Can you work these out from the model? Positions are in its coordinate system, mm. Round coordinates to 2 decimals unless told otherwise and drop trailing zeros. Write each loop counter-clockwise with the first axis right and the second up, starting at its lowest first coordinate (ties: lowest second). Pieces come first, ordered by that corner, then holes. Notation, with made-up numbers: (88.5, 36) - (140.5, 36) arc R35 ccw to (140.5, 75) - close; hole circle Ø3 at (66, 33.25). An arc over 180 degrees is marked (long way). One line per item, written item: value. Start each with the question number.
(1) I want a section at B-B on y = 0. List the corners of the cut face in (x, z) for me, plus the area to 3 significant figures.
(2) I want a section at D-D on z = -5. List the corners of the cut face in (x, y) for me.
(3) I want a section at A-A on z = 17.5. List the corners of the cut face in (x, y) for me, plus the area to 3 significant figures.
(4) I want a section at C-C on x = 0.9. List the corners of the cut face in (y, z) for me.
(5) I'm going to push flat-ended pins straight in: pin 1 Ø2 at (x, y) = (0, 0) entering from +Z; pin 2 Ø1.5 at (x, z) = (-0.5, 7) entering from -Y; pin 3 Ø1.2 at (x, y) = (0, -0.5) entering from -Z. Where does each tip first touch, or does it pass through?
(6) If I drill on L1, parallel to X at y = 0, z = 17.7; L2, parallel to Z at x = -0.4, y = 1; L3, parallel to Y at x = 0.8, z = 2.5, over which ranges is the centre line in solid material (lowest first)? Write a range as from..to.
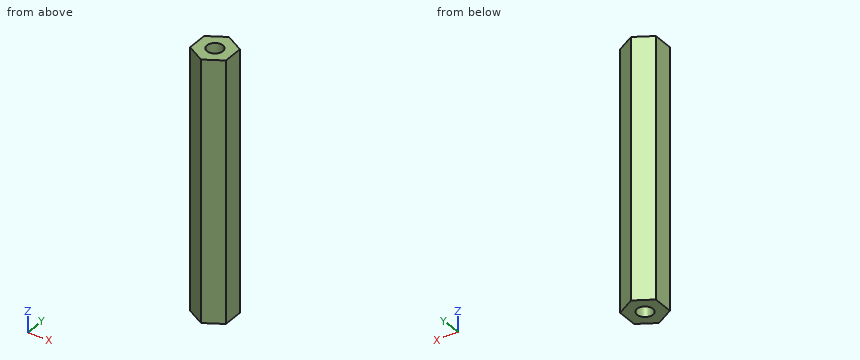
Autodesk Inventor part; units mm, degrees
ref_plane "YZ Plane" through (0, 0, 0) normal (1, 0, 0) x (0, 1, 0)
ref_plane "XZ Plane" through (0, 0, 0) normal (0, 1, 0) x (-1, 0, 0)
ref_plane "XY Plane" through (0, 0, 0) normal (0, 0, 1) x (1, 0, 0)
sketch "スケッチ1" plane through (0, 0, 0) normal (0, 0, 1) x (1, 0, 0)
  line L0 (2.75, 1.5877) -> (2.75, -1.5877)
  line L1 (2.75, -1.5877) -> (0, -3.1754)
  line L2 (0, -3.1754) -> (-2.75, -1.5877)
  line L3 (-2.75, -1.5877) -> (-2.75, 1.5877)
  line L4 (-2.75, 1.5877) -> (0, 3.1754)
  line L5 (0, 3.1754) -> (2.75, 1.5877)
  point P0 (0, 0)
  point P1 (0, 0)
  dimension "d0" = 5.5
extrude "押し出し1" add sketch "スケッチ1" along normal blind 20
sketch "スケッチ2" plane through (0, 0, 20) normal (0, 0, 1) x (1, 0, 0)
  point P0 (0, 0)
  point P1 (0, 0)
hole "穴1" at (0, 0, 20) direction (0, 0, -1) diameter 2.459 depth 6
mirror "ミラー1" about plane through (0, 0, 0) normal (0, 0, -1) of "押し出し1", "穴1"
properties part number "ASU-340" material "ステンレス鋼 AISI 304"
Established:
1. outline: (-2.75, -20) - (-1.23, -20) - (-1.23, -14) - (1.23, -14) - (1.23, -20) - (2.75, -20) - (2.75, 20) - (1.23, 20) - (1.23, 14) - (-1.23, 14) - (-1.23, 20) - (-2.75, 20) - close
1. area: 190 mm2
2. outline: (-2.75, -1.59) - (0, -3.18) - (2.75, -1.59) - (2.75, 1.59) - (0, 3.18) - (-2.75, 1.59) - close
3. outline: (-2.75, -1.59) - (0, -3.18) - (2.75, -1.59) - (2.75, 1.59) - (0, 3.18) - (-2.75, 1.59) - close; hole circle Ø2.46 at (0, 0)
3. area: 21.4 mm2
4. outline: (-2.66, -20) - (-0.84, -20) - (-0.84, -14) - (0.84, -14) - (0.84, -20) - (2.66, -20) - (2.66, 20) - (0.84, 20) - (0.84, 14) - (-0.84, 14) - (-0.84, 20) - (-2.66, 20) - close
5. pin 1: z = 14
5. pin 2: y = -3.18
5. pin 3: z = -14
6. L1: -2.75..-1.23, 1.23..2.75
6. L2: -14..14
6. L3: -2.71..2.71
